from build123d import *

# Parameters (mm, degrees)
F1_DEPTH = 1
F3_R     = 0.2
F5_R     = 2.5
F6_DEPTH = 8
F7_R     = 2.5


with BuildPart() as f1:
    # F0 (on Front) → F1 (new body)
    with BuildSketch(Plane.XZ):
        with BuildLine():
            ThreePointArc((-2.6, -1.2845232579), (2.9, 0), (-2.6, 1.2845232579))
            Line((-2.6, 1.2845232579), (-2.6, -1.2845232579))
        make_face()
    extrude(amount=F1_DEPTH)

    # F4: sweep along a path in F2
    with BuildLine(Plane.XY) as f4_path:
        Line((0, 0), (0, 12.5555443466))
        ThreePointArc((0, 12.5555443466), (-0.1464466094, 12.9090977372), (-0.5, 13.0555443466))
        Line((-0.5, 13.0555443466), (-4.480665084, 13.0555443466))
    # F3 (on Front) → F4 (sweep)
    with BuildSketch(Plane.XZ):
        with Locations((0, 1.27)):
            Circle(F3_R)
        with Locations((0, -1.27)):
            Circle(F3_R)
    sweep(path=f4_path.line)

    # F5 (on face) → F6 (join)
    with BuildSketch(Plane.XZ.offset(1)):
        Circle(F5_R)
    extrude(amount=F6_DEPTH)

    # F7
    f7_edges = [f1.edges().sort_by_distance(p)[0] for p in [
        (-2.5, -9, 0),
    ]]
    fillet(f7_edges, radius=F7_R)


solid = f1.part
Here's how the part is built. I have some questions about the finished solid (model axes, mm). A direction names the side the tool comes from. Give positions to 0.01 mm unless a question says otherwise; leave off trailing zeros. Write each loop counter-clockwise with the first axis right and the second up, starting at its lowest first coordinate (ties: lowest second). Pieces come first, ordered by that corner, then holes. Notation, with made-up numbers: (-20, 33) -> (39, 33) arc R18 cw to (39, 41) -> close; hole circle Ø1 at (48.5, -5.75). An arc over 180 degrees is marked (long way). Use one line per item in the form item = value. Start each with the question number.
1. Imagine slicing it at A-A on x = -0.75. List the corners of the cut face in (y, z) for me.
2. If I drill on L1, parallel to Z at x = 0, y = 3.5; L2, parallel to Y at x = -2.5, z = -0.9; L3, parallel to Z at x = -0.75, y = -2, over which ranges is the centre line in solid material (lowest first)?
3. On a 3-axis mill with a long thin cutter (end or side, diameter ignored), from which of +Z, -Z, +X, -X, +Y, -Y can I reach the whole of each face in a straight line? I mean faces 1 (the face through (-0.54, -3.71, -2.44)), 2 (the face through (-2.6, -0.5, 0)). Say none if no direction works.
4. Imagine slicing it at C-C on y = 11.5. List the corners of the cut face in (x, z) for me.
5. Imagine slicing it at B-B on z = 0. List the corners of the cut face in (x, y) for me, plus the area to 3 significant figures.
6. Will these pins go through, and if not, where does the flat tip stop? pin 1 Ø3 at (x, y) = (-0.5, 5.5) entering from +Z; pin 2 Ø0.5 at (y, z) = (-0.5, 0) entering from -X; pin 3 Ø1.5 at (y, z) = (1.5, 2) entering from +X.
7. Imagine slicing it at D-D on y = -0.75. List the corners of the cut face in (x, z) for me.
Entries:
q1.outline = (-6.5, -2.38) -> (-1, -2.38) -> (-1, -2.8) -> (0, -2.8) -> (0, 2.8) -> (-1, 2.8) -> (-1, 2.38) -> (-6.5, 2.38) arc R2.38 ccw to start; circle Ø0.4 at (13.06, -1.27); circle Ø0.4 at (13.06, 1.27)
q2.L1 = -1.47 to -1.07, 1.07 to 1.47
q2.L2 = -1 to 0
q2.L3 = -2.38 to 2.38
q3.face_1 = -Y
q3.face_2 = +Z, -Z, -X, -Y
q4.outline = circle Ø0.4 at (0, -1.27); circle Ø0.4 at (0, 1.27)
q5.outline = (-2.6, -1) -> (-2.5, -1) -> (-2.5, -6.5) arc R2.5 ccw to (2.5, -6.5) -> (2.5, -1) -> (2.9, -1) -> (2.9, 0) -> (-2.6, 0) -> close
q5.area = 42.8 mm²
q6.pin_1 = 1.47
q6.pin_2 = -2.6
q6.pin_3 = 0.2
q7.outline = (-2.6, -1.28) arc R2.9 ccw (long way) to (-2.6, 1.28) -> close
